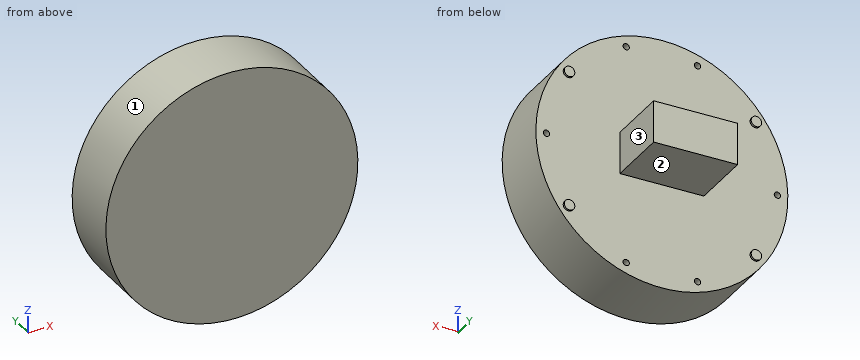
from build123d import *

# Parameters (mm, degrees)
SKETCH_1_R               = 60
EXTRUDE_1_DEPTH          = 30
SKETCH_2_R               = 1.5
CUT_EXTRUDE_1_DEPTH      = 5
PATTERN_CIRCULAR_1_COUNT = 10
SKETCH_3_W               = 40
SKETCH_3_H               = 20
EXTRUDE_2_DEPTH          = 30
SKETCH_5_R               = 2.5
EXTRUDE_4_DEPTH          = 1


with BuildPart() as part:
    # 草图1 → 凸台-拉伸1 (new body)
    with BuildSketch(Plane(origin=(0, 0, 0), x_dir=(1, 0, 0), z_dir=(0, 1, 0))):
        with Locations(Location((0, 0, 0), (0, 0, 270))):
            Circle(SKETCH_1_R)
    extrude(amount=EXTRUDE_1_DEPTH)

    # 草图2 → 切除-拉伸1 (cut)
    with BuildSketch(Plane(origin=(0, 30, 0), x_dir=(1, 0, 0), z_dir=(0, 1, 0))):
        with Locations(Location((55, 0, 0), (0, 0, 270))):
            Circle(SKETCH_2_R)
    cut_extrude_1 = extrude(amount=-CUT_EXTRUDE_1_DEPTH, mode=Mode.SUBTRACT)

    # 阵列(圆周)1: 切除-拉伸1 ×10 about axis
    pattern_circular_1_axis = Axis((0, 0, 0), (0, 1, 0))
    for i in range(1, PATTERN_CIRCULAR_1_COUNT):
        add(cut_extrude_1.rotate(pattern_circular_1_axis, i * 360 / PATTERN_CIRCULAR_1_COUNT), mode=Mode.SUBTRACT)

    # 草图3 → 凸台-拉伸2 (add)
    with BuildSketch(Plane(origin=(0, 30, 0), x_dir=(1, 0, 0), z_dir=(0, 1, 0))):
        Rectangle(SKETCH_3_W, SKETCH_3_H)
    extrude(amount=EXTRUDE_2_DEPTH)

    # 草图5 → 凸台-拉伸4 (add)
    with BuildSketch(Plane(origin=(0, 30, 0), x_dir=(1, 0, 0), z_dir=(0, 1, 0))):
        with Locations(Location((-44.495934691, 32.328188876, 0), (0, 0, 270))):
            Circle(SKETCH_5_R)
        with Locations(Location((44.495934691, -32.328188876, 0), (0, 0, 270))):
            Circle(SKETCH_5_R)
        with Locations(Location((44.495934691, 32.328188876, 0), (0, 0, 270))):
            Circle(SKETCH_5_R)
        with Locations(Location((-44.495934691, -32.328188876, 0), (0, 0, 270))):
            Circle(SKETCH_5_R)
    extrude(amount=EXTRUDE_4_DEPTH)


solid = part.part
Model file for the job. Use its own axes, mm. Face numbers are marked on the shaded views. A direction names the side the tool comes from. Give positions to 0.01 mm unless a question says otherwise; leave off trailing zeros. Write each loop counter-clockwise with the first axis right and the second up, starting at its lowest first coordinate (ties: lowest second). Pieces come first, ordered by that corner, then holes. Notation, with made-up numbers: (46.5, 61.25) -> (94.5, 61.25) arc R28 cw to (94.5, 90.25) -> close; hole circle Ø4 at (80.25, -37.75). An arc over 180 degrees is marked (long way). Write item = value, one per line.
(1) Slice it at D-D, the plane x = 55. Give the cut face in (y, z), then the cut area to 3 significant figures.
Determined:
outline = (0, -23.98) -> (30, -23.98) -> (30, -1.5) -> (25, -1.5) -> (25, 1.5) -> (30, 1.5) -> (30, 23.98) -> (0, 23.98) -> close
area = 1,420 mm2
(2) Slice it at C-C, the plane y = 5. Give the cut face in (x, z).
Determined:
outline = circle Ø120 at (0, 0)
(3) Tool access for the marked faces 1, 2 and 3: list every direction of +Z, -Z, +X, -X, +Y, -Y with a clear straight run to the whole face (end or side of a thin tool).
Determined:
face_1 = +Y, -Y
face_2 = -Z, +X, -X, +Y
face_3 = +Z, -Z, +X, +Y
(4) Probe line 1 along X through (y, z) = (26, 0); line 2 along Y through (x, z) = (24, 33); line 3 along Z through (x, y) = (16, 39). List the from-to ranges inside material, lowest first.
Determined:
line_1 = -60 to -56.5, -53.5 to 53.5, 56.5 to 60
line_2 = 0 to 30
line_3 = -10 to 10
(5) Flat gauge pins, fed straight in: P1, Ø4, axis at x = 45, z = 33, coming from the +Y side; P2, Ø3.5, axis at x = 17, z = 52.31, coming from the +Y side; P3, Ø2, axis at x = -7.5, y = 50.5, coming from the -Z side. Where does each tip first touch, or does it go through?
Determined:
P1 = 31
P2 = 30
P3 = -10
(6) Slice it at A-A, the plane x = 0. Give the cut face in (y, z).
Determined:
outline = (0, -60) -> (30, -60) -> (30, -10) -> (60, -10) -> (60, 10) -> (30, 10) -> (30, 60) -> (0, 60) -> close
(7) Slice it at B-B, the plane z = 0. Give the cut face in (x, y).
Determined:
outline = (-60, 0) -> (60, 0) -> (60, 30) -> (56.5, 30) -> (56.5, 25) -> (53.5, 25) -> (53.5, 30) -> (20, 30) -> (20, 60) -> (-20, 60) -> (-20, 30) -> (-53.5, 30) -> (-53.5, 25) -> (-56.5, 25) -> (-56.5, 30) -> (-60, 30) -> close
